Study the drawing (mm; zero at the part's minimum x, y, z) and answer. Give positions to 0.01 mm unless a question says otherwise; leave off trailing zeros. Loops run counter-clockwise (first coordinate to the right, second up) from the corner with the lowest first, then second, coordinate; pieces in that order, holes last. Notation, with made-up numbers: (59, 83.25) - (89, 83.25) arc R22 cw to (89, 95.25) - close; hole circle Ø4 at (-36.5, 84). An arc over 180 degrees is marked (long way). Write item = value, one per line. Start each with the question number.
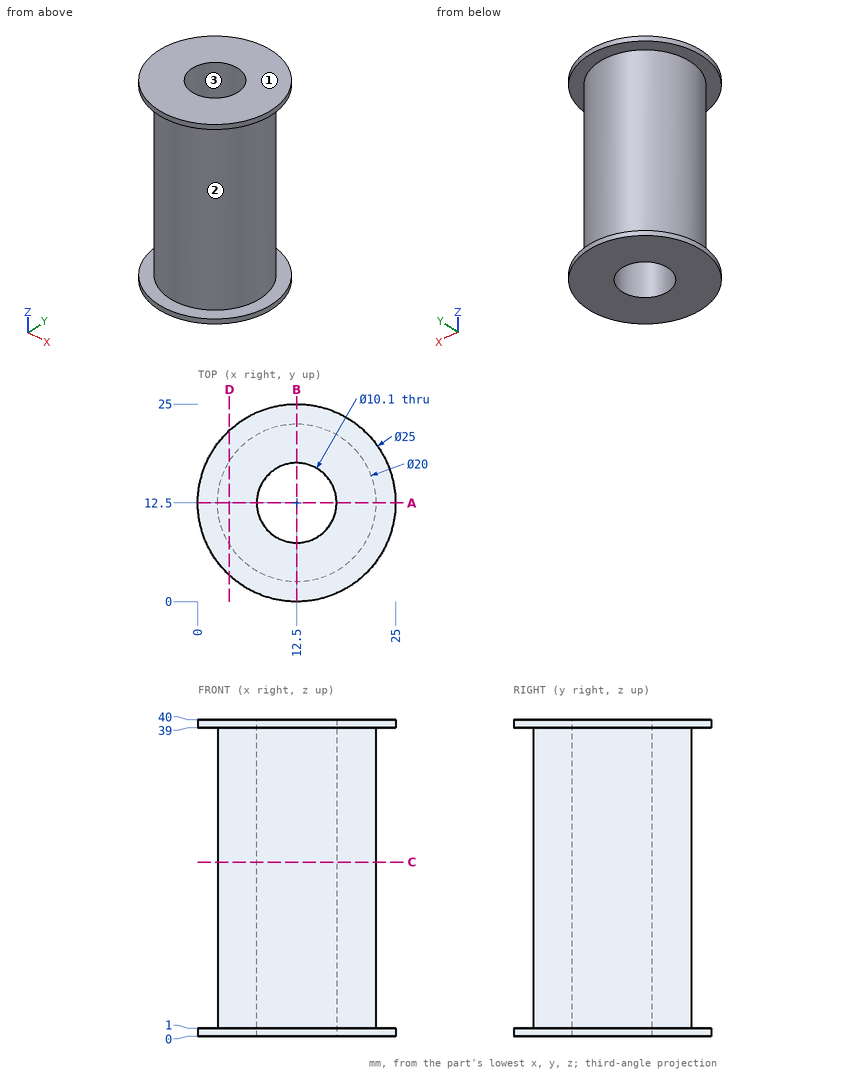
1. Given P1, Ø10, axis at x = 3.5, z = 22.5, coming from the +Y side; P2, Ø13, axis at x = 12.5, y = 12.5, coming from the +Z side; P3, Ø2, axis at x = 18, z = 18.5, coming from the +Y side; P4, Ø10, axis at y = 21.5, z = 33.5, coming from the -X side, each flat-ended and moving along its own axis, determine where each tip first touches the part or whether it passes through.
2. Consider line 1 along Z through (x, y) = (16.25, 24); line 2 along Y through (x, z) = (12.5, 13); line 3 along Y through (x, z) = (9.75, 32). Determine where each line is inside the solid, lowest interval first. Write a range as [from, to].
3. A cutting plane is placed at A-A on y = 12.5. Give the vertices of the cut face in (x, z), and give its area (3 significant figures).
4. A cutting plane is placed at D-D on x = 4. Give the vertices of the cut face in (y, z), and give its area (3 significant figures).
5. For a pull along X with two mould halves and no side action, classify the marked faces 1, 2 and 3 as released by +X, released by -X, zero draft, split by the parting line, or undercut.
6. A cutting plane is placed at C-C on z = 22. Give the vertices of the cut face in (x, y), and give its area (3 significant figures).
Reply:
q1.P1 = 21.67
q1.P2 = 40
q1.P3 = 21.43
q1.P4 = 3.33
q2.line_1 = [0, 1], [39, 40]
q2.line_2 = [2.5, 7.45], [17.55, 22.5]
q2.line_3 = [2.89, 8.26], [16.74, 22.11]
q3.outline = (0, 0) - (7.45, 0) - (7.45, 40) - (0, 40) - (0, 39) - (2.5, 39) - (2.5, 1) - (0, 1) - close; (17.55, 0) - (25, 0) - (25, 1) - (22.5, 1) - (22.5, 39) - (25, 39) - (25, 40) - (17.55, 40) - close
q3.area = 406 mm^2
q4.outline = (3.33, 0) - (21.67, 0) - (21.67, 1) - (17.77, 1) - (17.77, 39) - (21.67, 39) - (21.67, 40) - (3.33, 40) - (3.33, 39) - (7.23, 39) - (7.23, 1) - (3.33, 1) - close
q4.area = 437 mm^2
q5.face_1 = zero draft
q5.face_2 = split by the parting line
q5.face_3 = undercut
q6.outline = circle Ø20 at (12.5, 12.5); hole circle Ø10.1 at (12.5, 12.5)
q6.area = 234 mm^2
